Source: CAD feature listing. Evaluate the final solid. Frame: model axes, mm. A direction names the side the tool comes from. Coordinates: 2 decimals unless noted, no trailing zeros. Order: outer loops, then holes, each group sorted by start corner. A loop starts at its lowest first (then second) coordinate and runs counter-clockwise, first axis right, second up.
Solid Edge part; units mm, degrees
sketch "Sketch1" plane through (0, 0, 0) normal (0, -1, 0) x (1, 0, 0)
  circle A0 centre (0, 0) radius 12
extrude "Protrusion1" add sketch "Sketch1" against normal blind 14
sketch "Sketch2" plane through (0, 0, 0) normal (0, -1, 0) x (1, 0, 0)
  circle A0 centre (0, 0) radius 2
extrude "Cutout1" cut sketch "Sketch2" against normal up to next
sketch "Sketch3" plane through (0, 0, 0) normal (1, 0, 0) x (0, 1, 0)
  line L0 (2, 12) -> (4.7516, 3)
  line L1 (4.7516, 3) -> (9.2484, 3)
  line L2 (9.2484, 3) -> (12, 12)
  line L3 (12, 12) -> (2, 12)
revolve "RevolvedCutout1" cut sketch "Sketch3" angle 360 about axis through (0, 0, 0) along (0, 1, 0)
properties material "Steel"
1. Section query D-D, the plane y = 9.75. Output: boundary loops of the cut face in (x, z), plus the area to 3 significant figures.
2. Draft query along Z for faces 1 (the flat face through (0.2, 14, -2.5)), 2 (the cylindrical face through (0, 7, -3)), 3 (the cylindrical face through (0, 7, -2)). Return one class per face: +Z half, -Z half, draft (parallel to the pull), parting line (faces both ways), or undercut.
3. Section query B-B, the plane z = 0. Output: boundary loops of the cut face in (x, y), plus the area to 3 significant figures.
4. Section query C-C, the plane y = 8. Output: boundary loops of the cut face in (x, z).
5. Contact query for flat-ended pins moving along their axis: P1, Ø1.5, axis at x = -4, y = 2, coming from the +Z side; P2, Ø5, axis at y = 2, z = -4.5, coming from the +X side; P3, Ø1, axis at x = 2.5, y = 12.5, coming from the -Z side. Output: stop coordinate, or through.
6. Section query A-A, the plane x = 0. Output: boundary loops of the cut face in (y, z).
7. Access query for faces 4 (the cylindrical face through (-11.99, 12.99, 0.53)), 5 (the conical face through (1.07, 9.42, 3.4)). Directions: +Z, -Z, +X, -X, +Y, -Y. A direction counts if a zero-diameter tool reaches every point of the face in a straight line with its end or side. Return the directions, or none.
8. Material intervals for line 1 along Y through (x, z) = (11, 1.75); line 2 along Y through (x, z) = (6.5, 6); line 3 along X through (y, z) = (12.5, -9.75), sorted ascending.
Answer key:
1. outline: circle Ø9.28 at (0, 0); hole circle Ø4 at (0, 0)
1. area: 55.1 mm2
2. face 1: draft
2. face 2: parting line
2. face 3: undercut
3. outline: (-12, 0) - (-2, 0) - (-2, 14) - (-12, 14) - (-12, 12) - (-3, 9.25) - (-3, 4.75) - (-12, 2) - close; (2, 0) - (12, 0) - (12, 2) - (3, 4.75) - (3, 9.25) - (12, 12) - (12, 14) - (2, 14) - close
3. area: 150 mm2
4. outline: circle Ø6 at (0, 0); hole circle Ø4 at (0, 0)
5. P1: stops at z = 11.55
5. P2: stops at x = 11.83
5. P3: stops at z = -11.83
6. outline: (0, -12) - (2, -12) - (4.75, -3) - (9.25, -3) - (12, -12) - (14, -12) - (14, -2) - (0, -2) - close; (0, 2) - (14, 2) - (14, 12) - (12, 12) - (9.25, 3) - (4.75, 3) - (2, 12) - (0, 12) - close
7. face 4: +Y, -Y
7. face 5: none
8. line 1: y = 0 to 2.26, 11.74 to 14
8. line 2: y = 0 to 2.96, 11.04 to 14
8. line 3: x = -7 to 7
